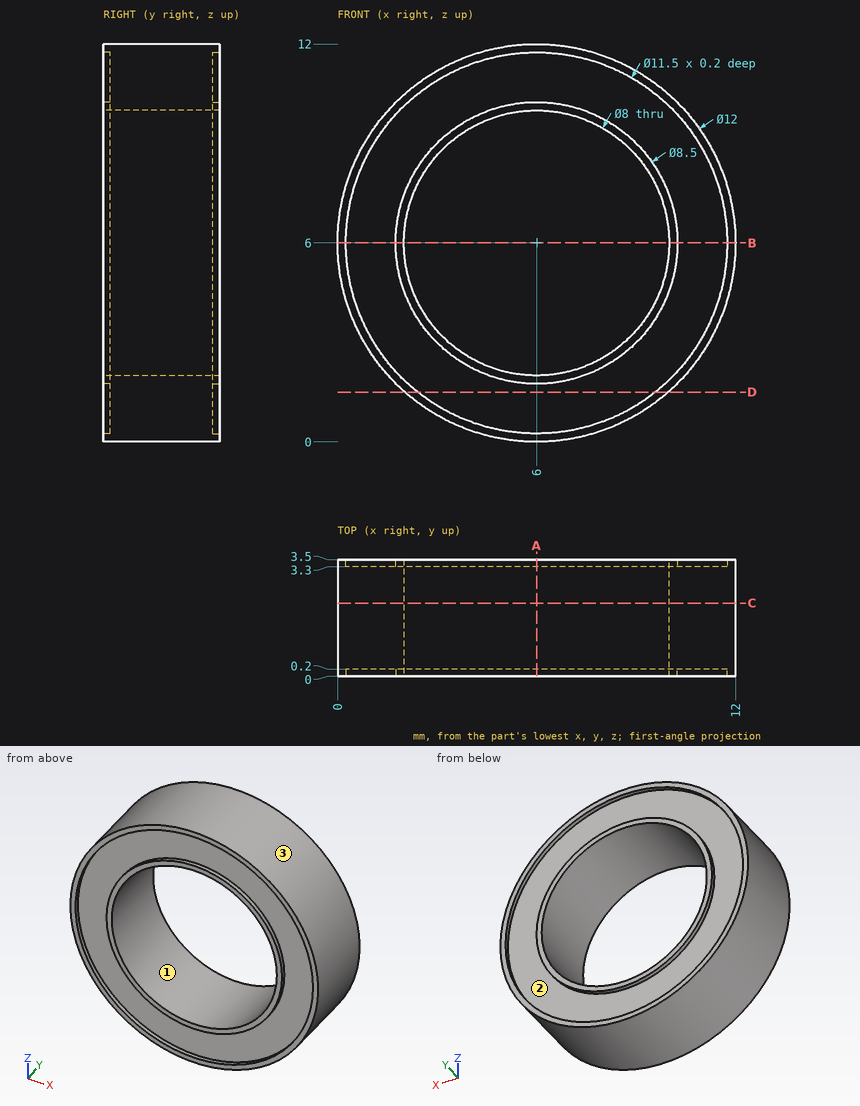
Answer from the drawing. Dimensions are ordinates in mm from the lowest x, y and z of the part. Give positions to 0.01 mm unless a question says otherwise; leave off trailing zeros. Order: outer loops, then holes, each group sorted by start corner. A loop starts at its lowest first (then second) coordinate and runs counter-clockwise, first axis right, second up.
(1) Straight lines are drawn through the part: L1, parallel to X at y = 0.15, z = 6; L2, parallel to Z at x = 6, y = 1. For each, find the intervals that lie inside material, in ascending order.
(2) Given pin 1 (1 mm diameter, centred on y = 1, z = 4.5, fed in from -X), flat-ended and moving along its own axis, determine where the tip first touches the part or whether it passes through.
(3) Find section D-D (z = 1.5). Give the vertices of the cut face in (x, y).
(4) For a pull along X with two mould halves and no side action, classify the marked faces 1, 2 and 3 as released by +X, released by -X, zero draft, split by the parting line, or undercut.
(5) Find section A-A (x = 6). Give the vertices of the cut face in (y, z), plus the area to 3 significant figures.
(6) Find section C-C (y = 2.2). Give the vertices of the cut face in (x, z), plus the area to 3 significant figures.
(7) Find section B-B (z = 6). Give the vertices of the cut face in (x, y), plus the area to 3 significant figures.
Result sheet:
1. L1: x = 0 to 0.25, 1.75 to 2, 10 to 10.25, 11.75 to 12
1. L2: z = 0 to 2, 10 to 12
2. pin 1: stops at x = 0.08
3. outline: (2.03, 0) - (2.42, 0) - (2.42, 0.2) - (9.58, 0.2) - (9.58, 0) - (9.97, 0) - (9.97, 3.5) - (9.58, 3.5) - (9.58, 3.3) - (2.42, 3.3) - (2.42, 3.5) - (2.03, 3.5) - close
4. face 1: undercut
4. face 2: undercut
4. face 3: split by the parting line
5. outline: (0, 0) - (3.5, 0) - (3.5, 0.25) - (3.3, 0.25) - (3.3, 1.75) - (3.5, 1.75) - (3.5, 2) - (0, 2) - (0, 1.75) - (0.2, 1.75) - (0.2, 0.25) - (0, 0.25) - close; (0, 10) - (3.5, 10) - (3.5, 10.25) - (3.3, 10.25) - (3.3, 11.75) - (3.5, 11.75) - (3.5, 12) - (0, 12) - (0, 11.75) - (0.2, 11.75) - (0.2, 10.25) - (0, 10.25) - close
5. area: 12.8 mm2
6. outline: circle Ø12 at (6, 6); hole circle Ø8 at (6, 6)
6. area: 62.8 mm2
7. outline: (0, 0) - (0.25, 0) - (0.25, 0.2) - (1.75, 0.2) - (1.75, 0) - (2, 0) - (2, 3.5) - (1.75, 3.5) - (1.75, 3.3) - (0.25, 3.3) - (0.25, 3.5) - (0, 3.5) - close; (10, 0) - (10.25, 0) - (10.25, 0.2) - (11.75, 0.2) - (11.75, 0) - (12, 0) - (12, 3.5) - (11.75, 3.5) - (11.75, 3.3) - (10.25, 3.3) - (10.25, 3.5) - (10, 3.5) - close
7. area: 12.8 mm2
